from build123d import *
from OCP.BRepFilletAPI import BRepFilletAPI_MakeChamfer

# Parameters (mm, degrees)
BOSS_EXTRUDE1_DEPTH = 20
SKETCH3_W           = 42.34282297
SKETCH3_H           = 14
CUT_EXTRUDE1_DEPTH  = 10
CUT_EXTRUDE2_DEPTH  = 14
SKETCH2_R           = 2.2
CUT_EXTRUDE3_DEPTH  = 6
CHAMFER1_SIZE       = 1
CHAMFER1_SIZE2      = 0.9011492
CHAMFER1_SIZE2_2    = 1.140658854


with BuildPart() as part:
    # Sketch1 → Boss-Extrude1 (new body)
    with BuildSketch(Plane.XY):
        Polygon((0, 58.251961434), (0, 0), (50, 0), (50, 52.38682507), align=None)
    extrude(amount=BOSS_EXTRUDE1_DEPTH)

    # Sketch3 → Cut-Extrude1 (cut)
    with BuildSketch(Plane(origin=(6.041343432, 51.502156617, 0), x_dir=(0.9931902315046269, -0.11650392286865593, 0), z_dir=(0.11650392286865592, 0.9931902315046268, 0))):
        with Locations((18.384829463, -10)):
            Rectangle(SKETCH3_W, SKETCH3_H)
    extrude(amount=-CUT_EXTRUDE1_DEPTH, mode=Mode.SUBTRACT)

    # Sketch4 → Cut-Extrude2 (cut)
    with BuildSketch(Plane.XY.offset(3)):
        Polygon((2.10869816, 41.894902039), (2.10869816, 0), (44.163176308, 0), (44.163176308, 36.961797057), align=None)
    extrude(amount=CUT_EXTRUDE2_DEPTH, mode=Mode.SUBTRACT)

    # Sketch2 → Cut-Extrude3 (cut)
    with BuildSketch(Plane(origin=(6.740366969, 57.461298006, 0), x_dir=(0.9931902315046269, -0.11650392286865593, 0), z_dir=(0.11650392286865592, 0.9931902315046268, 0))):
        with Locations(Location((3.213417978, -10, 0), (0, 0, 180))):
            Circle(SKETCH2_R)
        with Locations(Location((33.556240948, -10, 0), (0, 0, 180))):
            Circle(SKETCH2_R)
    extrude(amount=-CUT_EXTRUDE3_DEPTH, mode=Mode.SUBTRACT)

    # Chamfer1: one chamfer whose edges measure the first distance from different faces: ONE call of the kernel's chamfer builder (chamfer() names one face for all edges)
    chamfer1_edges_1 = [part.edges().sort_by_distance(p)[0] for p in [
        (25, 55.319393252, 20),
        (0, 29.125980717, 20),
        (0, 29.125980717, 0),
        (25, 55.319393252, 0),
        (50, 26.193412535, 0),
        (50, 26.193412535, 20),
    ]]
    chamfer1_edges_2 = [part.edges().sort_by_distance(p)[0] for p in [
        (0, 58.251961434, 10),
    ]]
    chamfer1_side_2 = [part.faces().sort_by_distance(p)[0] for p in [
        (25, 55.319393252, 10),
    ]]
    chamfer1_edges_3 = [part.edges().sort_by_distance(p)[0] for p in [
        (50, 52.38682507, 10),
    ]]
    chamfer1_side_3 = [part.faces().sort_by_distance(p)[0] for p in [
        (50, 26.193412535, 10),
    ]]
    chamfer1 = BRepFilletAPI_MakeChamfer(part.part.solid().wrapped)
    for e in chamfer1_edges_1:
        chamfer1.Add(CHAMFER1_SIZE, e.wrapped)
    for e in chamfer1_edges_2:
        chamfer1.Add(CHAMFER1_SIZE, CHAMFER1_SIZE2, e.wrapped, chamfer1_side_2[0].wrapped)  # the first distance lies on this face
    for e in chamfer1_edges_3:
        chamfer1.Add(CHAMFER1_SIZE, CHAMFER1_SIZE2_2, e.wrapped, chamfer1_side_3[0].wrapped)  # the first distance lies on this face
    add(Compound.cast(chamfer1.Shape()), mode=Mode.REPLACE)


solid = part.part
Can you work these out from the model? Positions are in its coordinate system, mm. A direction names the side the tool comes from. Round coordinates to 2 decimals unless told otherwise and drop trailing zeros. Order: outer loops, then holes, each group sorted by start corner. A loop starts at its lowest first (then second) coordinate and runs counter-clockwise, first axis right, second up. Notation, with made-up numbers: M 7.25,67.25 L 46.25,67.25 A10 cw 46.25,71.25 Z; hole C 48.5,82 d2. An arc over 180 degrees is marked long. Use a Markdown table: item, result.
1) Imagine slicing it at D-D (z = 15.75). List the corners of the cut face in (x, y) for me, then the cut area to 3 significant figures.
Geometry says:
| item | result |
|---|---|
| outline | M 0,0 L 2.11,0 L 2.11,41.89 L 3.27,51.83 L 45.33,46.89 L 44.16,36.96 L 44.16,0 L 50,0 L 50,51.39 L 48.87,52.52 L 0.99,58.14 L 0,57.35 Z |
| area | 683 mm² |
2) If I drill on line 1 along Z through (x, y) = (24, 26); line 2 along X through (y, z) = (6.5, 15.75); line 3 along X through (y, z) = (41, 5.75), over which ranges is the centre line in solid material (lowest first)?
Geometry says:
| item | result |
|---|---|
| line 1 | z = 0 to 3, 17 to 20 |
| line 2 | x = 0 to 2.11, 44.16 to 50 |
| line 3 | x = 0 to 2.11, 44.64 to 50 |
3) If we mould it in two halves opening along X, with no side actions, what happens to faces 1 (the face through (23, 26, 3)), 2 (the face through (28.6, 0, 2.5)), 3 (the face through (25.265, 55.288, 9.874))? For each: +X half, -X half, draft (parallel to the pull), parting line (faces both ways), or undercut.
Geometry says:
| item | result |
|---|---|
| face 1 | undercut |
| face 2 | draft |
| face 3 | +X half |
4) On a 3-axis mill with a long thin cutter (end or side, diameter ignored), from which of +Z, -Z, +X, -X, +Y, -Y can I reach the whole of each face in a straight line? I mean faces 4 (the face through (44.754, 41.997, 10.098)), 5 (the face through (25, 29, 0)), 6 (the face through (2.109, 21, 10)). Say none if no direction works.
Geometry says:
| item | result |
|---|---|
| face 4 | none |
| face 5 | -Z, +X, -X, +Y, -Y |
| face 6 | -Y |
5) Imagine slicing it at B-B (z = 8.5). List the corners of the cut face in (x, y) for me, then the cut area to 3 significant figures.
Geometry says:
| item | result |
|---|---|
| outline | M 0,0 L 2.11,0 L 2.11,41.89 L 3.27,51.83 L 7.63,51.32 L 8.33,57.27 L 0.99,58.14 L 0,57.35 Z; M 10.83,50.94 L 37.77,47.78 L 38.47,53.74 L 11.53,56.9 Z; M 40.97,47.41 L 45.33,46.89 L 44.16,36.96 L 44.16,0 L 50,0 L 50,51.39 L 48.87,52.52 L 41.67,53.36 Z |
| area | 645 mm² |
6) I'm going to push flat-ended pins straight in: P1, Ø2, axis at x = 16, z = 7.5, coming from the -Y side; P2, Ø2, axis at x = 28.5, z = 5.5, coming from the -Y side; P3, Ø1, axis at x = 30, z = 9.5, coming from the +Y side; P4, Ø12, axis at x = 40, z = 9.5, coming from the -Y side. Where does each tip first touch, or does it pass through?
Geometry says:
| item | result |
|---|---|
| P1 | stops at y = 50.22 |
| P2 | stops at y = 48.75 |
| P3 | stops at y = 54.79 |
| P4 | stops at y = 0 |
7) Imagine slicing it at A-A (y = 11). List the corners of the cut face in (x, z) for me.
Geometry says:
| item | result |
|---|---|
| outline | M 0,1 L 1,0 L 49,0 L 50,1 L 50,19 L 49,20 L 1,20 L 0,19 Z; hole M 2.11,3 L 44.16,3 L 44.16,17 L 2.11,17 Z |
8) Imagine slicing it at C-C (x = 15). List the corners of the cut face in (y, z) for me, then the cut area to 3 significant figures.
Geometry says:
| item | result |
|---|---|
| outline | M 0,0 L 55.49,0 L 56.49,1 L 56.49,19 L 55.49,20 L 0,20 L 0,17 L 50.45,17 L 50.45,3 L 0,3 Z |
| area | 423 mm² |
